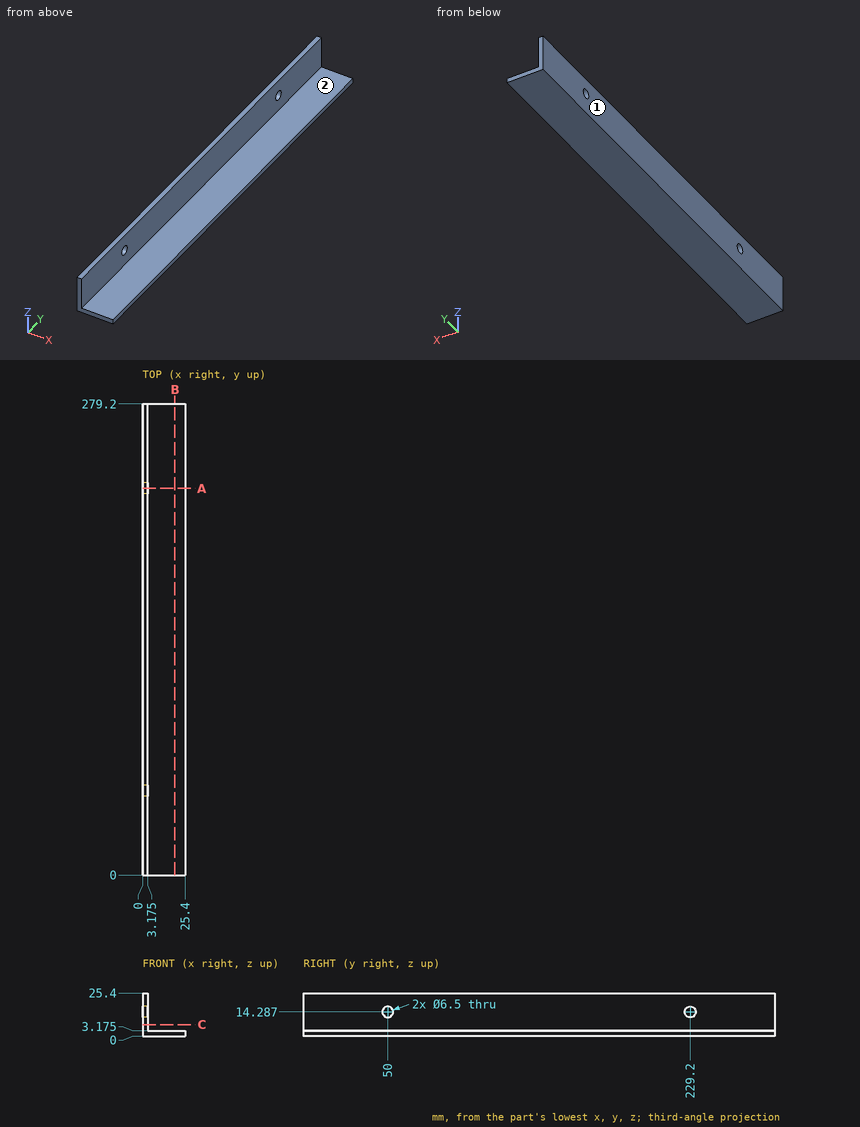
Check sheet for the drawn part. Datum: minimum x, y, z corner. Units: mm. A direction names the side the tool comes from. Coordinates: 2 decimals unless noted, no trailing zeros. Order: outer loops, then holes, each group sorted by start corner. A loop starts at its lowest first (then second) coordinate and runs counter-clockwise, first axis right, second up. Notation, with made-up numbers: M -23,-19.75 L 27,-19.75 A19 ccw 27,9.25 Z; hole C 30.25,11 d6. An arc over 180 degrees is marked long. One line per question, with ' | ' between items. Start each with the question number.
Item 1: Gauge pin test, flat ends, axial feed: pin 1 (6 mm diameter, centred on y = 50, z = 14.29, fed in from +X); pin 2 (3 mm diameter, centred on y = 102, z = 14.5, fed in from +X) (1 decimal); pin 3 (11 mm diameter, centred on x = 11, y = 105, fed in from +Z) (1 decimal). Record the tip position at first contact, or that the pin passes through.
Item 2: Cross-section at B-B on x = 19.25. Enter the section's corners in (y, z) (1 decimal).
Item 3: Cross-section at C-C on z = 6.75. Enter the section's corners in (x, y) (1 decimal).
Item 4: Material ranges on L1, parallel to Z at x = 2.5, y = 229.2; L2, parallel to Y at x = 1.5, z = 11.5 (1 decimal); L3, parallel to Y at x = 3, z = 15.5 (1 decimal), recorded low to high. Write a range as [from, to].
Item 5: Set-up check for the marked faces 1 and 2: record each of +Z, -Z, +X, -X, +Y, -Y from which the full face is reachable in a straight line by a thin tool's end or side.
Item 6: Cross-section at A-A on y = 229.2. Enter the section's corners in (x, z) (1 decimal).
Findings:
1) pin 1: passes through | pin 2: stops at x = 3.2 | pin 3: stops at z = 3.2
2) outline: M 0,0 L 279.2,0 L 279.2,3.2 L 0,3.2 Z
3) outline: M 0,0 L 3.2,0 L 3.2,279.2 L 0,279.2 Z
4) L1: z = [0, 11.04], [17.54, 25.4] | L2: y = [0, 48.3], [51.7, 227.5], [230.9, 279.2] | L3: y = [0, 47], [53, 226.2], [232.2, 279.2]
5) face 1: +Z, -Z, -X, +Y, -Y | face 2: +Z, +X, +Y, -Y
6) outline: M 0,0 L 25.4,0 L 25.4,3.2 L 3.2,3.2 L 3.2,11 L 0,11 Z; M 0,17.5 L 3.2,17.5 L 3.2,25.4 L 0,25.4 Z
